Could you check a few things on this model? Use its own coordinates, in mm. A direction names the side the tool comes from. Round coordinates to 2 decimals unless told otherwise and drop trailing zeros. Loops run counter-clockwise (first coordinate to the right, second up) from the corner with the lowest first, then second, coordinate; pieces in that order, holes last. Notation, with made-up numbers: (75, 63.5) - (126, 63.5) arc R12 ccw to (126, 80.5) - close; hole circle Ø6 at (19, -35). An arc over 180 degrees is marked (long way). Use one line per item in the form item = value.
Autodesk Inventor part; units mm, degrees
ref_plane "YZ Plane" through (0, 0, 0) normal (1, 0, 0) x (0, 1, 0)
ref_plane "XZ Plane" through (0, 0, 0) normal (0, 1, 0) x (-1, 0, 0)
ref_plane "XY Plane" through (0, 0, 0) normal (0, 0, 1) x (1, 0, 0)
sketch "Эскиз1" plane through (0, 0, 0) normal (0, 1, 0) x (-1, 0, 0)
  line L0 (34, 53) -> (-34, 53)
  line L1 (-34, 53) -> (-34, -53)
  line L2 (-34, -53) -> (34, -53)
  line L3 (34, -53) -> (34, 53)
  line L4 (34, 53) -> (-34, -53) construction
  line L5 (-34, 53) -> (34, -53) construction
  line L6 (38, 57) -> (-38, 57)
  line L7 (-38, 57) -> (-38, -57)
  line L8 (-38, -57) -> (38, -57)
  line L9 (38, -57) -> (38, 57)
  point P0 (0, 0)
  dimension "d1" = 68
  dimension "d2" = 106
  dimension "d3" = 4
extrude "Выдавливание1" add sketch "Эскиз1" along normal blind 2 contours L3 L2 L1 L0
extrude "Выдавливание2" add sketch "Эскиз1" along normal blind 7
sketch "Эскиз2" plane through (0, 7, 0) normal (0, 1, 0) x (1, 0, 0)
  line L0 (34, -53) -> (-34, -53)
  line L1 (34, 53) -> (-34, 53)
  line L2 (-34, 53) -> (-34, -53)
  line L3 (-34, -53) -> (34, -53)
  line L4 (34, -53) -> (34, 53)
  line L5 (34, 53) -> (-34, -53) construction
  line L6 (-34, 53) -> (34, -53) construction
  line L7 (-34, -53) -> (-34, -50)
  line L8 (-34, -50) -> (34, -50)
  line L9 (-34, 53) -> (34, 53)
  line L10 (-34, 53) -> (-34, 50)
  line L11 (-34, 50) -> (34, 50)
  line L12 (34, 53) -> (34, -53)
  line L13 (34, -50) -> (27, -50)
  line L14 (27, -50) -> (27, 50)
  line L15 (-34, 50) -> (-31, 50)
  line L16 (-31, 50) -> (-31, -50)
  point P0 (0, 0)
  dimension "d8" = 3
  dimension "d9" = 3
  dimension "d10" = 7
  dimension "d11" = 3
extrude "Выдавливание3" add sketch "Эскиз2" against normal blind 2 contours L0 L2 L8 L4 | L8 L14 L11 L4 | L2 L11 L16 L8 | L11 L2 L1 L4
sketch "Эскиз3" plane through (38, 0, 57) normal (1, 0, 0) x (0, 0, -1)
  line L0 (114, 0) -> (0, 0)
  line L1 (0, 0) -> (16, 0)
  line L2 (16, 0) -> (16, 7)
  line L3 (114, 7) -> (0, 7)
  line L4 (114, 0) -> (114, 7)
  line L5 (114, 0) -> (98, 0)
  line L6 (98, 0) -> (98, 7)
  line L7 (98, 7) -> (114, 7)
  line L8 (114, 7) -> (114, 0)
  line L9 (0, 0) -> (0, 7)
  line L10 (0, 7) -> (16, 7)
  line L11 (15, 6) -> (15, 1)
  line L12 (15, 1) -> (1, 1)
  line L13 (1, 1) -> (1, 6)
  line L14 (1, 6) -> (15, 6)
  line L15 (99, 6) -> (99, 1)
  line L16 (99, 1) -> (113, 1)
  line L17 (113, 1) -> (113, 6)
  line L18 (113, 6) -> (99, 6)
  line L19 (16, 0) -> (17, 0)
  line L20 (17, 0) -> (17, 2)
  line L21 (98, 0) -> (97, 0)
  line L22 (97, 0) -> (97, 2)
  line L23 (96.5, 2) -> (17.5, 2)
  line L24 (17, 2.5) -> (17, 3.5)
  line L25 (17.5, 4) -> (96.5, 4)
  line L26 (97, 3.5) -> (97, 2.5)
  line L27 (110, 2) -> (4, 2)
  arc A0 (17.5, 4) -> (17, 3.5) centre (17.5, 3.5) ccw
  arc A1 (17, 2.5) -> (17.5, 2) centre (17.5, 2.5) ccw
  arc A2 (97, 3.5) -> (96.5, 4) centre (96.5, 3.5) ccw
  arc A3 (96.5, 2) -> (97, 2.5) centre (96.5, 2.5) ccw
  point P0 (57, 0)
  point P1 (17, 4)
  dimension "d14" = 16
  dimension "d15" = 16
  dimension "d16" = 1
  dimension "d17" = 1
  dimension "d18" = 1
  dimension "d19" = 2
  dimension "d20" = 1
  dimension "d21" = 2
  dimension "d22" = 2
  dimension "d23" = 0.5
extrude "Выдавливание4" cut sketch "Эскиз3" against normal blind 3 contours L23 A1 L24 A0 L25 A2 L26 A3
extrude "Выдавливание5" add sketch "Эскиз3" along normal blind 1 contours L15 L18 L17 L16 | L11 L12 L13 L14
sketch "Эскиз4" plane through (38, 0, -57) normal (0, 0, -1) x (-1, 0, 0)
  line L0 (0, 0) -> (76, 0)
  line L1 (76, 0) -> (76, 2)
  line L2 (76, 0) -> (76, 7)
  line L3 (72, 2) -> (72, 5)
  line L4 (76, 2) -> (72, 2)
  line L5 (72, 2) -> (72, 5)
  line L6 (72, 5) -> (76, 5)
  line L7 (76, 5) -> (76, 2)
  line L8 (72, 5) -> (72, 6)
  line L9 (72, 6) -> (74, 6)
  line L10 (74, 6) -> (74, 5)
  line L11 (74, 2) -> (74, 1)
  line L12 (74, 1) -> (72, 1)
  line L13 (72, 1) -> (72, 2)
  point P0 (38, 0)
  dimension "d28" = 2
  dimension "d29" = 1
  dimension "d30" = 2
  dimension "d31" = 1
extrude "Выдавливание6" cut sketch "Эскиз4" against normal blind 120
sketch "Эскиз5" plane through (38, 1, 56) normal (0, 0, 1) x (1, 0, 0)
  line L0 (1, 5) -> (1, 0)
  line L1 (1, 0) -> (1, 2.5)
  line L2 (1, 2.5) -> (4.5, 2.5)
  circle A0 centre (4.5, 2.5) radius 3.5
  arc A1 (2.75, -0.5311) -> (1, 0) centre (0.4167, -5.0709) ccw
  arc A2 (1, 5) -> (2.6628, 5.479) centre (0.4389, 10.0731) ccw
  circle A3 centre (4.5, 2.5) radius 2
  point P0 (-38, -1)
  dimension "d34" = 2.5
  dimension "d36" = 3.5
  dimension "d37" = 5.104
  dimension "d38" = 4
extrude "Выдавливание7" add sketch "Эскиз5" against normal blind 112
sketch "Эскиз6" plane through (38, 1, 42) normal (0, 0, -1) x (-1, 0, 0)
  line L0 (0, 5) -> (-1, 5)
  line L1 (-1, 5) -> (-1, 8.1758)
  line L2 (-1, 8.1758) -> (-10.78, 8.3268)
  line L3 (-10.78, 8.3268) -> (-10.1005, -3.8271)
  line L4 (-10.1005, -3.8271) -> (-1.8469, -2.418)
  line L5 (-1.8469, -2.418) -> (-1, -0.011)
  line L6 (-1, -0.011) -> (-1, 5)
  point P0 (38, -1)
extrude "Выдавливание8" cut sketch "Эскиз6" along normal blind 84
sketch "Эскиз7" plane through (0, 0, 0) normal (0, -1, 0) x (1, 0, 0)
  circle A0 centre (0, 0) radius 34
  circle A1 centre (0, 0) radius 32.5
  line L0 (-17, -57.0311) -> (17, -57.0311)
  line L1 (-17, -57.0311) -> (-17, -35.0999)
  line L2 (-38, 57) -> (38, 57)
  line L3 (17, 57) -> (-17, 57)
  arc A2 (17, 35.0999) -> (-17, 35.0999) centre (0, 0) ccw
  arc A3 (-17, -35.0999) -> (17, -35.0999) centre (0, 0) ccw
  line L4 (-17, 35.0999) -> (-17, 57)
  line L5 (17, 35.0999) -> (17, 57)
  line L6 (17, -57.0311) -> (17, -35.0999)
  line L7 (-15.4, -37.5659) -> (-15.4, -55.4311)
  line L8 (15.4, -55.4311) -> (15.4, -37.5659)
  arc A4 (-15.4, -37.5659) -> (15.4, -37.5659) centre (0, 0) ccw
  line L9 (15.4, 55.4) -> (15.4, 37.5659)
  arc A5 (15.4, 37.5659) -> (-15.4, 37.5659) centre (0, 0) ccw
  line L10 (-15.4, 37.5659) -> (-15.4, 55.4)
  line L11 (-15.4, -55.4311) -> (-15.4, -57.0311)
  line L12 (15.4, -55.4311) -> (15.4, -57.0311)
  line L13 (-15.4, 55.4) -> (-15.4, 57)
  line L14 (15.4, 55.4) -> (15.4, 57)
  dimension "d43" = 65
  dimension "d51" = 1.6
  dimension "d52" = 1.6
extrude "Выдавливание9" add sketch "Эскиз7" along normal blind 1 contours A0 | L1 A3 L6 L0 L12 L8 A4 L7 L11 | L2 L13 L10 A5 L9 L14 L5 A2 L4
sketch "Эскиз8" plane through (-38, 7, 57) normal (0, 0, 1) x (1, 0, 0)
  line L0 (21, -7) -> (21, -8)
  line L1 (21, -8) -> (21, 0)
  line L2 (76, 0) -> (0, 0)
  line L3 (55, -8) -> (21, -8)
  line L4 (21, -8) -> (22.6, -8)
  line L5 (22.6, -8) -> (22.6, 0)
  line L6 (22.6, 0) -> (21, 0)
  line L7 (53.4, -7) -> (53.4, -8)
  line L8 (53.4, -8) -> (53.4, 0)
  line L9 (53.4, 0) -> (55, 0)
  line L10 (55, 0) -> (55, -8)
  line L11 (55, -8) -> (53.4, -8)
  point P0 (38, -7)
  dimension "d55" = 1.6
  dimension "d56" = 1.6
extrude "Выдавливание10" add sketch "Эскиз8" along normal blind 1 contours L1 L2 L5 L3 L0 | L7 L8 L2 L10 L3
sketch "Эскиз9" plane through (38, 7, -57) normal (0, 0, -1) x (-1, 0, 0)
  line L0 (55, -7) -> (55, -8)
  line L1 (55, -8) -> (55, 0)
  line L2 (55, 0) -> (53.4, 0)
  line L3 (53.4, -7) -> (53.4, -8)
  line L4 (53.4, 0) -> (53.4, -8)
  line L5 (53.4, -8) -> (55, -8)
  line L6 (22.6, -7) -> (22.6, -8)
  line L7 (22.6, -8) -> (22.6, 0)
  line L8 (22.6, 0) -> (21, 0)
  line L9 (21, 0) -> (21, -8)
  line L10 (21, -8) -> (22.6, -8)
  point P0 (38, -7)
  dimension "d59" = 8
  dimension "d60" = 1.6
  dimension "d61" = 1.6
extrude "Выдавливание11" add sketch "Эскиз9" along normal blind 1
sketch "Эскиз10" plane through (0, 7, 0) normal (0, 1, 0) x (1, 0, 0)
  line L0 (-15.4, -58) -> (-17, -58)
  line L1 (-17, -58) -> (-17, -50)
  line L2 (27, -50) -> (-31, -50)
  line L3 (-15.4, -57) -> (-15.4, -58)
  line L4 (-15.4, -58) -> (-17, -58)
  line L5 (-15.4, -58) -> (-15.4, -50)
  line L6 (-15.4, -50) -> (-17, -50)
  line L7 (15.4, -58) -> (15.4, -50)
  line L8 (15.4, -50) -> (17, -50)
  line L9 (17, -35.0999) -> (17, -58)
  line L10 (17, -58) -> (15.4, -58)
  line L11 (17, -58) -> (17, -50)
  line L12 (-17, 58) -> (-15.4, 58)
  line L13 (-17, 58) -> (-17, 50)
  line L14 (-17, 50) -> (-15.4, 50)
  line L15 (-15.4, 50) -> (-15.4, 58)
  line L16 (-15.4, 58) -> (-17, 58)
  line L17 (15.4, 58) -> (15.4, 50)
  line L18 (15.4, 50) -> (17, 50)
  line L19 (17, 58) -> (17, 50)
  line L20 (15.4, 58) -> (17, 58)
  point P0 (0, 0)
  dimension "d64" = 8
extrude "Выдавливание12" add sketch "Эскиз10" along normal blind 1
properties part number "Дета2ль1"
1. If we section it at C-C, the plane x = 0: Write out the boundary of the cut face in (y, z), plus the area to 3 significant figures.
Solution:
outline = (-1, -40.6) - (0, -40.6) - (0, -57) - (7, -57) - (7, -50) - (5, -50) - (5, -53) - (2, -53) - (2, 53) - (5, 53) - (5, 50) - (7, 50) - (7, 57) - (0, 57) - (0, 40.6) - (-1, 40.6) - (-1, 39) - (0, 39) - (0, 34) - (-1, 34) - (-1, 32.5) - (0, 32.5) - (0, -32.5) - (-1, -32.5) - (-1, -34) - (0, -34) - (0, -39) - (-1, -39) - close
area = 286 mm^2
2. Please list where these lines run through material, in increasing order: line 1 along Z through (x, y) = (12, 4); line 2 along Z through (x, y) = (16, 5.75); line 3 along Y through (x, z) = (-16.5, -51).
Solution:
line_1 = -57 to -53, 53 to 57
line_2 = -58 to -50, 50 to 58
line_3 = -1 to 2, 5 to 8
3. We'd pull the mould along Z, two halves only. Please class faces 1 (the face through (28, 5, -4)), 2 (the face through (15.4, -0.5, -50.8)), 3 (the face through (40, 3, 56)): +Z half, -Z half, draft (parallel to the pull), parting line (faces both ways), or undercut.
Solution:
face_1 = undercut
face_2 = draft
face_3 = +Z half
4. If we section it at B-B, the plane x = 42.5: Write out the boundary of the cut face in (y, z).
Solution:
outline = (0, -56) - (1.5, -56) - (1.5, -42) - (0, -42) - close; (0, 42) - (1.5, 42) - (1.5, 56) - (0, 56) - close; (5.5, -56) - (7, -56) - (7, -42) - (5.5, -42) - close; (5.5, 42) - (7, 42) - (7, 56) - (5.5, 56) - close
5. For P1, Ø3, axis at x = 6.5, y = 5.5, coming from the -Z side; P2, Ø1.5, axis at x = -19.5, y = 0.5, coming from the +Z side; P3, Ø2, axis at y = 6, z = -46, coming from the +X side; P4, Ø2.5, axis at y = 3, z = 49.5, coming from the +X side, each with a flat end and sliding along its axis, tell me the tip position at first contact or that it passes through.
Solution:
P1 = -57
P2 = 57
P3 = 45.66
P4 = 46
6. On a 3-axis mill with a long thin cutter (end or side, diameter ignored), from which of +Z, -Z, +X, -X, +Y, -Y can I reach the whole of each face in a straight line? I mean faces 4 (the face through (0, 0, -47)), 5 (the face through (0, 7, 54)), 6 (the face through (40, 4, 42)), 7 (the face through (0, 0, 47)). Say none if no direction works.
Solution:
face_4 = -Z, -Y
face_5 = +Z, -Z, +Y
face_6 = +X, +Y, -Y
face_7 = +Z, -Y
